Autodesk Inventor part; units mm, degrees
ref_plane "YZ Plane" through (0, 0, 0) normal (1, 0, 0) x (0, 1, 0)
ref_plane "XZ Plane" through (0, 0, 0) normal (0, 1, 0) x (-1, 0, 0)
ref_plane "XY Plane" through (0, 0, 0) normal (0, 0, 1) x (1, 0, 0)
sketch "Sketch1" plane through (0, 0, 0) normal (0, 1, 0) x (-1, 0, 0)
  circle A0 centre (0, 0) radius 1.15
  circle A1 centre (0, 0) radius 2.5
  dimension "d0" = 2.3
  dimension "d1" = 5
extrude "Extrusion1" add sketch "Sketch1" along normal blind 9
sketch "Sketch2" plane through (0, 0, 0) normal (0, 0, 1) x (1, 0, 0)
  line L0 (2.5, 9) -> (-2.5, 9)
  line L1 (2.5, 0) -> (-2.5, 0)
  line L2 (-2.5, 0) -> (-2.5, 9)
  line L3 (-2.5, 7) -> (2.5173, 7)
  line L4 (2.5, 9) -> (-2.5, 9)
  line L5 (0, 9) -> (0, 0)
  circle A0 centre (0, 4.9) radius 2.1
  dimension "d4" = 2
  dimension "d5" = 4.2
extrude "Extrusion2" cut sketch "Sketch2" along normal blind 12 contours A0 L5 | L5 A0
sketch "Sketch3" plane through (0, 0, 0) normal (1, 0, 0) x (0, 1, 0)
  line L0 (9, -2.5) -> (9, 2.5)
  line L1 (0, -2.5) -> (0, 2.5)
  line L2 (0, 2.5) -> (9, 2.5)
  line L3 (7, 2.5) -> (7, -2.525)
  line L4 (9, 1.15) -> (9, -1.15)
  line L5 (9, 0) -> (0, 0)
  circle A0 centre (4.9, 0) radius 2.1
  point P0 (4.9, 1.3565)
  dimension "d8" = 2
  dimension "d9" = 4.2
extrude "Extrusion3" cut sketch "Sketch3" along normal up to next contours A0 L5 | L5 A0
properties part number "motor_shaft_adapter" material "ABS Plastic"
The listing builds one solid part. Answer for the finished solid, in the listing's coordinates (mm). A direction names the side the tool comes from. Coordinates: 2 decimals unless noted, no trailing zeros. Loops run counter-clockwise (first coordinate to the right, second up) from the corner with the lowest first, then second, coordinate; pieces in that order, holes last. Notation, with made-up numbers: (51.25, 66.25) - (90.25, 66.25) arc R28 cw to (90.25, 89.25) - close; hole circle Ø11 at (-40, -8.5). An arc over 180 degrees is marked (long way). Write item = value, one per line.
1) Each of these flat-tipped pins is pushed along its axis until it touches: P1, Ø3, axis at x = -0.5, z = -1, coming from the -Y side; P2, Ø2, axis at x = 2, y = 4, coming from the +Z side; P3, Ø0.8, axis at x = -1.5, y = 4.5, coming from the +Z side. Where does it stop, or does it pass through?
Responses:
P1 = 0
P2 = 2.12
P3 = 0
2) Section A-A (z = 1.95) is taken. Determine the outline of the cut face in (x, y).
Responses:
outline = (-1.56, 0) - (1.56, 0) - (1.56, 3.5) arc R2.1 cw to (-1.56, 3.5) - close; (-1.56, 6.3) arc R2.1 cw to (1.56, 6.3) - (1.56, 9) - (-1.56, 9) - close
3) Section D-D (z = -1.6) is taken. Determine the outline of the cut face in (x, y), plus the area to 3 significant figures.
Responses:
outline = (-1.92, 0) - (1.92, 0) - (1.92, 3.54) - (0, 3.54) - (0, 6.26) - (1.92, 6.26) - (1.92, 9) - (-1.92, 9) - close
area = 29.4 mm^2
4) Section B-B (x = -1) is taken. Determine the outline of the cut face in (y, z), plus the area to 3 significant figures.
Responses:
outline = (0, -2.29) - (9, -2.29) - (9, -0.57) - (0, -0.57) - close; (0, 0.57) - (3.05, 0.57) - (3.05, 2.29) - (0, 2.29) - close; (6.75, 0.57) - (9, 0.57) - (9, 2.29) - (6.75, 2.29) - close
area = 24.7 mm^2
5) Determine the mould class of faces 1 (the face through (-1.5, 4.9, 0)), 2 (the face through (-1.097, 4.437, -0.345)), 3 (the face through (-1.34, 4.44, -2.11)), 4 (the face through (0, 4.9, -1.5)) for opening direction X: pulls with the +X half, pulls with the -X half, needs draft (parallel to the pull), parting line crosses it, or undercut.
Responses:
face_1 = needs draft
face_2 = undercut
face_3 = parting line crosses it
face_4 = pulls with the +X half
6) Which of the six approach directions +Z, -Z, +X, -X, +Y, -Y give full straight-line access (tool end or side, diameter ignored) to faces 5 (the face through (-2.1, 4.82, 0.95)), 6 (the face through (0.95, 4.98, -2.1)), 7 (the face through (-1, 0, -1))?
Responses:
face_5 = +Z
face_6 = +X
face_7 = +Z, -Z, +X, -X, -Y
7) Section C-C (y = 8.25) is taken. Determine the outline of the cut face in (x, z).
Responses:
outline = circle Ø5 at (0, 0); hole circle Ø2.3 at (0, 0)
8) Find the intervals of material crossed by line 1 along Y through (x, z) = (0, 1.4); line 2 along X through (y, z) = (1.75, -0.75); line 3 along X through (y, z) = (3.5, 1.65), in increasing order.
Responses:
line_1 = 0 to 2.8, 7 to 9
line_2 = -2.38 to -0.87, 0.87 to 2.38
line_3 = -1.88 to -1.57, 1.57 to 1.88
